The drawing under review shows one solid part. Ordinate dimensions are in mm from its lowest x, y, z. Give positions to 0.01 mm unless a question says otherwise; leave off trailing zeros. Write each loop counter-clockwise with the first axis right and the second up, starting at its lowest first coordinate (ties: lowest second). Pieces come first, ordered by that corner, then holes. Notation, with made-up numbers: (27, -34.5) -> (84, -34.5) arc R29 cw to (84, -14.5) -> close; hole circle Ø2 at (-32.75, 81.5). An arc over 180 degrees is marked (long way). Answer as a JSON object with one key per item and string values.
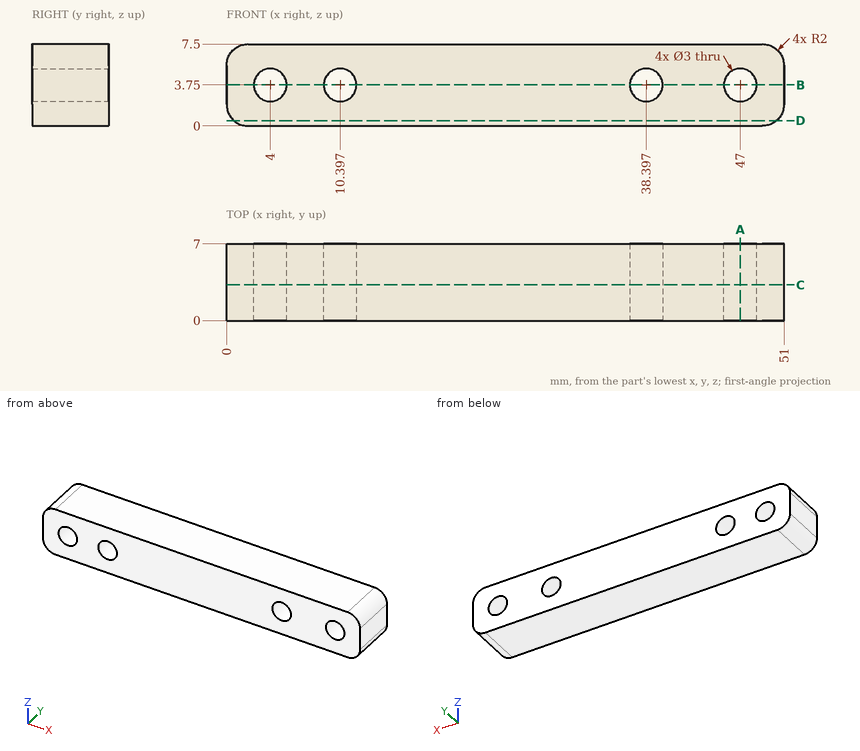
(1) For line 1 along Z through (x, y) = (47, 2.25); line 2 along X through (y, z) = (5.5, 4); line 3 along X through (y, z) = (0.5, 3), list the stretches that pass through material, from the lowest coordinate up.
Here are the results:
{"line 1": "z = 0 to 2.25, 5.25 to 7.5", "line 2": "x = 0 to 2.52, 5.48 to 8.92, 11.88 to 36.92, 39.88 to 45.52, 48.48 to 51", "line 3": "x = 0 to 2.7, 5.3 to 9.1, 11.7 to 37.1, 39.7 to 45.7, 48.3 to 51"}
(2) We need section D-D, the plane z = 0.5. State the section outline as (x, y) points.
Here are the results:
{"outline": "(0.68, 0) -> (50.32, 0) -> (50.32, 7) -> (0.68, 7) -> close"}
(3) We need section B-B, the plane z = 3.75. State the section outline as (x, y) points, then the cut area to 3 significant figures.
Here are the results:
{"outline": "(0, 0) -> (2.5, 0) -> (2.5, 7) -> (0, 7) -> close; (5.5, 0) -> (8.9, 0) -> (8.9, 7) -> (5.5, 7) -> close; (11.9, 0) -> (36.9, 0) -> (36.9, 7) -> (11.9, 7) -> close; (39.9, 0) -> (45.5, 0) -> (45.5, 7) -> (39.9, 7) -> close; (48.5, 0) -> (51, 0) -> (51, 7) -> (48.5, 7) -> close", "area": "273 mm²"}
(4) We need section C-C, the plane y = 3.25. State the section outline as (x, z) points, then the cut area to 3 significant figures.
Here are the results:
{"outline": "(0, 2) arc R2 ccw to (2, 0) -> (49, 0) arc R2 ccw to (51, 2) -> (51, 5.5) arc R2 ccw to (49, 7.5) -> (2, 7.5) arc R2 ccw to (0, 5.5) -> close; hole circle Ø3 at (4, 3.75); hole circle Ø3 at (10.4, 3.75); hole circle Ø3 at (38.4, 3.75); hole circle Ø3 at (47, 3.75)", "area": "351 mm²"}
(5) We need section A-A, the plane x = 47. State the section outline as (y, z) points.
Here are the results:
{"outline": "(0, 0) -> (7, 0) -> (7, 2.25) -> (0, 2.25) -> close; (0, 5.25) -> (7, 5.25) -> (7, 7.5) -> (0, 7.5) -> close"}
